```python
from build123d import *

# Parameters (mm, degrees)
F1_DEPTH = 5


with BuildPart() as f1:
    # F0 (on Front) → F1 (new body)
    with BuildSketch(Plane.XZ):
        Polygon((0, 0), (0, 70), (-24.521741, 70), (-24.521741, 60), (-29.521741, 60), (-29.521741, 50), (-24.521741, 50), (-24.521741, 40), (-29.521741, 40), (-29.521741, 30), (-24.521741, 30), (-24.521741, 20), (-29.521741, 20), (-29.521741, 10), (-24.521741, 10), (-24.521741, 0), align=None)
        Polygon((24.521741, 70), (0, 70), (0, 0), (24.521741, 0), (24.521741, 10), (29.521741, 10), (29.521741, 20), (24.521741, 20), (24.521741, 30), (29.521741, 30), (29.521741, 40), (24.521741, 40), (24.521741, 50), (29.521741, 50), (29.521741, 60), (24.521741, 60), align=None)
    extrude(amount=F1_DEPTH)


solid = f1.part
```
The listing builds one solid part. Answer for the finished solid, in the listing's coordinates (mm). A direction names the side the tool comes from. Round coordinates to 2 decimals unless told otherwise and drop trailing zeros. Loops run counter-clockwise (first coordinate to the right, second up) from the corner with the lowest first, then second, coordinate; pieces in that order, holes last.
1) For a pull along Z with two mould halves and no side action, classify faces 1 (the face through (27, -2, 30)), 2 (the face through (0, -5, 35)), 3 (the face through (24.522, -2, 25)), 4 (the face through (0, -2, 0)) as released by +Z, released by -Z, zero draft, split by the parting line, or undercut.
Outcome:
face 1: undercut
face 2: zero draft
face 3: undercut
face 4: released by -Z
2) Consider line 1 (X direction, y = -4.15, z = 21). Determine where the line is inside the solid, lowest interval first.
Outcome:
line 1: x = -24.52 to 24.52
3) For faces 5 (the face through (24.522, -2, 45)), 6 (the face through (-24.522, -2, 65)), 7 (the face through (27, -2, 10)), determine the directions among +Z, -Z, +X, -X, +Y, -Y from which every point of the face is accessible in a straight line to the end or side of a thin tool.
Outcome:
face 5: +X, +Y, -Y
face 6: +Z, -X, +Y, -Y
face 7: -Z, +X, +Y, -Y
4) A cutting plane is placed at B-B on z = 45.5. Determine the outline of the cut face in (x, y), plus the area to 3 significant figures.
Outcome:
outline: (-24.52, -5) - (24.52, -5) - (24.52, 0) - (-24.52, 0) - close
area: 245 mm2
5) Given P1, Ø1.5, axis at x = -27, y = -2, coming from the -Z side; P2, Ø2.5, axis at y = -1.5, z = 3, coming from the -X side; P3, Ø2.5, axis at x = -26, y = -2.5, coming from the +Z side, each flat-ended and moving along its own axis, determine where each tip first touches the part or whether it passes through.
Outcome:
P1: stops at z = 10
P2: stops at x = -24.52
P3: stops at z = 60
6) A cutting plane is placed at A-A on y = -1.1. Determine the outline of the cut face in (x, z), plus the area to 3 significant figures.
Outcome:
outline: (-29.52, 10) - (-24.52, 10) - (-24.52, 0) - (24.52, 0) - (24.52, 10) - (29.52, 10) - (29.52, 20) - (24.52, 20) - (24.52, 30) - (29.52, 30) - (29.52, 40) - (24.52, 40) - (24.52, 50) - (29.52, 50) - (29.52, 60) - (24.52, 60) - (24.52, 70) - (-24.52, 70) - (-24.52, 60) - (-29.52, 60) - (-29.52, 50) - (-24.52, 50) - (-24.52, 40) - (-29.52, 40) - (-29.52, 30) - (-24.52, 30) - (-24.52, 20) - (-29.52, 20) - close
area: 3,730 mm2
